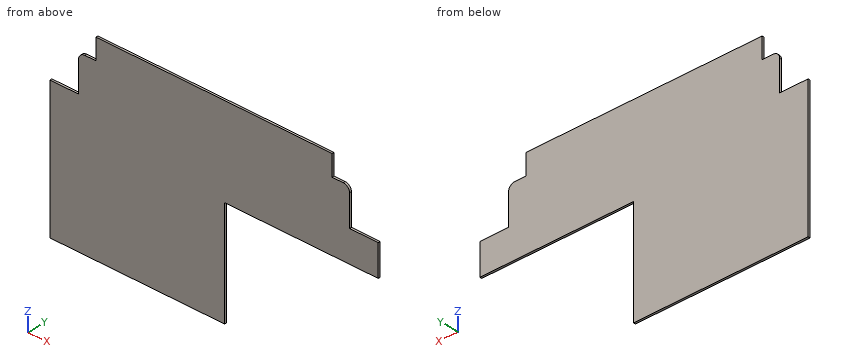
from build123d import *

# Parameters (mm, degrees)
CROQUIS1_W              = 250
CROQUIS1_H              = 250
SALIENTE_EXTRUIR1_DEPTH = 3
CROQUIS2_W              = 250
CROQUIS2_H              = 3
SALIENTE_EXTRUIR2_DEPTH = 3
CROQUIS3_W              = 220
CROQUIS3_H              = 99.34
SALIENTE_EXTRUIR4_DEPTH = 3
CROQUIS4_W              = 41
CROQUIS4_H              = 52
CORTAR_EXTRUIR1_DEPTH   = 3
CORTAR_EXTRUIR2_DEPTH   = 3
CROQUIS6_W              = 339
CROQUIS6_H              = 30
SALIENTE_EXTRUIR5_DEPTH = 3
CORTAR_EXTRUIR3_DEPTH   = 3
CROQUIS8_W              = 1
CROQUIS8_H              = 30
CORTAR_EXTRUIR4_DEPTH   = 10
CROQUIS10_W             = 41
CROQUIS10_H             = 1
CORTAR_EXTRUIR5_DEPTH   = 3


with BuildPart() as part:
    # Croquis1 → Saliente-Extruir1 (new body)
    with BuildSketch(Plane(origin=(0, 0, 0), x_dir=(1, 0, 0), z_dir=(0, 1, 0))):
        Rectangle(CROQUIS1_W, CROQUIS1_H)
    extrude(amount=SALIENTE_EXTRUIR1_DEPTH)

    # Croquis2 → Saliente-Extruir2 (add)
    with BuildSketch(Plane(origin=(0, 3, 0), x_dir=(1, 0, 0), z_dir=(0, 1, 0))):
        with Locations((0, 126.5)):
            Rectangle(CROQUIS2_W, CROQUIS2_H)
    extrude(amount=-SALIENTE_EXTRUIR2_DEPTH)

    # Croquis3 → Saliente-Extruir4 (add)
    with BuildSketch(Plane(origin=(0, 3, 0), x_dir=(1, 0, 0), z_dir=(0, 1, 0))):
        with Locations((235, -75.33)):
            Rectangle(CROQUIS3_W, CROQUIS3_H)
    extrude(amount=-SALIENTE_EXTRUIR4_DEPTH)

    # Croquis4 → Cortar-Extruir1 (cut)
    with BuildSketch(Plane(origin=(0, 3, 0), x_dir=(1, 0, 0), z_dir=(0, 1, 0))):
        with Locations((-104.5, -99)):
            Rectangle(CROQUIS4_W, CROQUIS4_H)
    extrude(amount=-CORTAR_EXTRUIR1_DEPTH, mode=Mode.SUBTRACT)

    # Croquis5 → Cortar-Extruir2 (cut)
    with BuildSketch(Plane(origin=(0, 3, 0), x_dir=(1, 0, 0), z_dir=(0, 1, 0))):
        with BuildLine():
            Line((-84, -116), (-84, -125))
            Line((-84, -125), (-75, -125))
            ThreePointArc((-75, -125), (-81.363961031, -122.363961031), (-84, -116))
        make_face()
    extrude(amount=-CORTAR_EXTRUIR2_DEPTH, mode=Mode.SUBTRACT)

    # Croquis6 → Saliente-Extruir5 (add)
    with BuildSketch(Plane(origin=(0, 3, 0), x_dir=(1, 0, 0), z_dir=(0, 1, 0))):
        with Locations((110.5, -140)):
            Rectangle(CROQUIS6_W, CROQUIS6_H)
    extrude(amount=-SALIENTE_EXTRUIR5_DEPTH)

    # Croquis7 → Cortar-Extruir3 (cut)
    with BuildSketch(Plane(origin=(0, 3, 0), x_dir=(1, 0, 0), z_dir=(0, 1, 0))):
        with BuildLine():
            Line((345, -72), (304, -72))
            Line((304, -72), (304, -116))
            ThreePointArc((304, -116), (301.363961031, -122.363961031), (295, -125))
            Line((295, -125), (345, -125))
            Line((345, -125), (345, -72))
        make_face()
    extrude(amount=-CORTAR_EXTRUIR3_DEPTH, mode=Mode.SUBTRACT)

    # Croquis8 → Cortar-Extruir4 (cut)
    with BuildSketch(Plane(origin=(0, 3, 0), x_dir=(1, 0, 0), z_dir=(0, 1, 0))):
        with Locations((279.5, -140)):
            Rectangle(CROQUIS8_W, CROQUIS8_H)
    extrude(amount=-CORTAR_EXTRUIR4_DEPTH, mode=Mode.SUBTRACT)

    # Croquis10 → Cortar-Extruir5 (cut)
    with BuildSketch(Plane(origin=(0, 3, 0), x_dir=(1, 0, 0), z_dir=(0, 1, 0))):
        with Locations((-104.5, -72.5)):
            Rectangle(CROQUIS10_W, CROQUIS10_H)
        with Locations((324.5, -71.5)):
            Rectangle(CROQUIS10_W, CROQUIS10_H)
    extrude(amount=-CORTAR_EXTRUIR5_DEPTH, mode=Mode.SUBTRACT)


solid = part.part
Verification items for the finished model (mm, model axes). Coordinates: 2 decimals unless noted, no trailing zeros. Loops run counter-clockwise (first coordinate to the right, second up) from the corner with the lowest first, then second, coordinate; pieces in that order, holes last. Notation, with made-up numbers: (-19.75, 11.5) -> (8.25, 11.5) arc R26 ccw to (8.25, 48.5) -> close; hole circle Ø5 at (58, 1). An arc over 180 degrees is marked (long way). Answer as CSV lines item,"result".
1) Thickness scan on L1, parallel to X at y = 0.85, z = -47.5; L2, parallel to Z at x = -90.5, y = 2.1; L3, parallel to X at y = 1.25, z = 84. Record the ranges inside material, lowest first. Write a range as from..to.
Found:
L1,"x = -125..125"
L2,"z = -128..72"
L3,"x = -84..304"
2) Depth check by flat-ended pin: pin 1 (1.5 mm diameter, centred on x = 283.5, y = 1, fed in from +Z); pin 2 (0.9 mm diameter, centred on x = 332.5, y = 2, fed in from +Z); pin 3 (0.9 mm diameter, centred on y = 1, z = 103.5, fed in from +X); pin 4 (4 mm diameter, centred on x = 222, z = 48, fed in from -Y). Enter the tip coordinate at first touch or a pass-through.
Found:
pin 1,"stops at z = 125"
pin 2,"stops at z = 71"
pin 3,"stops at x = 304"
pin 4,"stops at y = 0"
3) Cross-section at A-A, the plane y = 1.8. Record the cut outline in (x, z).
Found:
outline,"(-125, -128) -> (125, -128) -> (125, 25.66) -> (345, 25.66) -> (345, 71) -> (304, 71) -> (304, 116) arc R9 ccw to (295, 125) -> (279, 125) -> (279, 155) -> (-59, 155) -> (-59, 125) -> (-75, 125) arc R9 ccw to (-84, 116) -> (-84, 72) -> (-125, 72) -> close"
4) Cross-section at B-B, the plane z = -78. Record the cut outline in (x, y).
Found:
outline,"(-125, 0) -> (125, 0) -> (125, 3) -> (-125, 3) -> close"
5) Cross-section at C-C, the plane x = 150. Record the cut outline in (y, z).
Found:
outline,"(0, 25.66) -> (3, 25.66) -> (3, 155) -> (0, 155) -> close"
